Here's how the part is built. I have some questions about the finished solid (model axes, mm). A direction names the side the tool comes from. Coordinates: 2 decimals unless noted, no trailing zeros. Write each loop counter-clockwise with the first axis right and the second up, starting at its lowest first coordinate (ties: lowest second). Pieces come first, ordered by that corner, then holes. Notation, with made-up numbers: (78, -22.5) -> (128, -22.5) arc R18 cw to (128, -18.5) -> close; hole circle Ø7 at (28, 48). An arc over 180 degrees is marked (long way). Put each result on its own line as item: value. Start each with the question number.
Item 1: On a 3-axis mill with a long thin cutter (end or side, diameter ignored), from which of +Z, -Z, +X, -X, +Y, -Y can I reach the whole of each face in a straight line? I mean faces 5 (the face through (43, -45, 44)), 6 (the face through (-40, 47, 44)), 7 (the face through (46, -46, 85)), 8 (the face through (-47, -40, 44)), 9 (the face through (11.3, 50, 4.5)). Say none if no direction works.
Item 2: I need wall thicknesses on line 1 (X direction, y = -44, z = 68); line 2 (X direction, y = -45.5, z = 81). Which ranges of each line are inside material? Lowest first, please. Write a range as [from, to].
Item 3: For pin 1 (12 mm diameter, centred on x = -30, y = -20.5, fed in from -Z), with a flat end and sliding along its axis, tell me the tip position at first contact or that it passes through.
Item 4: I want a section at B-B, the plane y = -19. List the corners of the cut face in (x, z) for me, then the cut area to 3 significant figures.
Item 5: I want a section at A-A, the plane z = 59.5. List the corners of the cut face in (x, y) for me.
Item 6: If we mould it in two halves opening along X, with no side actions, what happens to faces 1 (the face through (-45, 42, 44)), 2 (the face through (-48, 40, 44)), 3 (the face through (45, 43, 44)), 4 (the face through (50, -11.3, 4.5))? For each: released by +X, released by -X, zero draft, split by the parting line, or undercut.
from build123d import *

# Parameters (mm, degrees)
F0_W     = 100
F0_H     = 100
F1_DEPTH = 5
F3_DEPTH = 80


with BuildPart() as f1:
    # F0 (on Top) → F1 (new body)
    with BuildSketch(Plane.XY):
        Rectangle(F0_W, F0_H)
    extrude(amount=F1_DEPTH)

    # F2 (on face) → F3 (join)
    with BuildSketch(Plane.XY.offset(5)):
        Polygon((-40, 45), (-40, 50), (-50, 50), (-50, 40), (-45, 40), (-45, 45), align=None)
        Polygon((40, 45), (45, 45), (45, 40), (50, 40), (50, 50), (40, 50), align=None)
        Polygon((-40, -45), (-45, -45), (-45, -40), (-50, -40), (-50, -50), (-40, -50), align=None)
        Polygon((50, -40), (45, -40), (45, -45), (40, -45), (40, -50), (50, -50), align=None)
    extrude(amount=F3_DEPTH)


solid = f1.part
Calculated:
1. face 5: +Z
1. face 6: +Z, +Y, -Y
1. face 7: +Z, +X, -X, +Y, -Y
1. face 8: +Z, +X, -X
1. face 9: +Z, -Z, +X, -X, +Y
2. line 1: x = [-50, -45], [45, 50]
2. line 2: x = [-50, -40], [40, 50]
3. pin 1: stops at z = 0
4. outline: (-50, 0) -> (50, 0) -> (50, 5) -> (-50, 5) -> close
4. area: 500 mm2
5. outline: (-50, -50) -> (-40, -50) -> (-40, -45) -> (-45, -45) -> (-45, -40) -> (-50, -40) -> close; (-50, 40) -> (-45, 40) -> (-45, 45) -> (-40, 45) -> (-40, 50) -> (-50, 50) -> close; (40, -50) -> (50, -50) -> (50, -40) -> (45, -40) -> (45, -45) -> (40, -45) -> close; (40, 45) -> (45, 45) -> (45, 40) -> (50, 40) -> (50, 50) -> (40, 50) -> close
6. face 1: undercut
6. face 2: zero draft
6. face 3: undercut
6. face 4: released by +X
